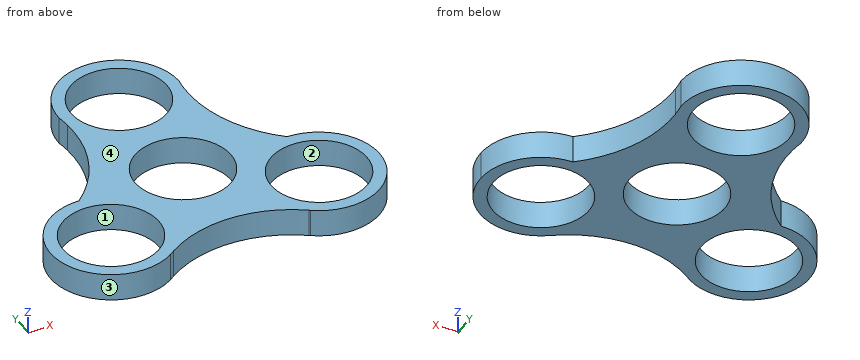
```python
from build123d import *

# Parameters (mm, degrees)
F0_R     = 11.049
F1_DEPTH = 6.35


with BuildPart() as f1:
    # F0 (on Top) → F1 (new body)
    with BuildSketch(Plane.XY):
        with BuildLine():
            ThreePointArc((24.1897099326, -0.0073616562), (15.9969747128, 11.215659094), (13.6372355628, 24.909042032))
            ThreePointArc((13.6372355628, 24.909042032), (-0.0068169573, 13.9700016632), (-13.6401871082, 24.9223526296))
            ThreePointArc((-13.6401871082, 24.9223526296), (-16.005456745, 11.2251220811), (-24.2066450876, 0.00241586))
            ThreePointArc((-24.2066450876, 0.00241586), (-14.3283633544, -4.0893024068), (-10.2366450876, -13.96758414))
            ThreePointArc((-10.2366450876, -13.96758414), (-11.6035855434, -19.9945062505), (-15.4369013691, -24.8419804502))
            ThreePointArc((-15.4369013691, -24.8419804502), (0.2894413219, -20.0870403352), (15.8966507841, -25.2195175864))
            ThreePointArc((15.8966507841, -25.2195175864), (10.9191820919, -9.6122739335), (24.1897099326, -0.0073616562))
        make_face()
        Circle(F0_R, mode=Mode.SUBTRACT)
        with BuildLine():
            ThreePointArc((-10.2366450876, -13.96758414), (-14.3283633544, -4.0893024068), (-24.2066450876, 0.00241586))
            ThreePointArc((-24.2066450876, 0.00241586), (-37.6059680769, -17.9196776899), (-16.6253454512, -25.7015006142))
            ThreePointArc((-16.6253454512, -25.7015006142), (-16.0368970517, -25.263757415), (-15.4369013691, -24.8419804502))
            ThreePointArc((-15.4369013691, -24.8419804502), (-11.6035855434, -19.9945062505), (-10.2366450876, -13.96758414))
        make_face()
        with Locations((-24.2066450876, -13.96758414)):
            Circle(F0_R, mode=Mode.SUBTRACT)
        with BuildLine():
            ThreePointArc((38.1597099326, -13.9773616562), (34.0679916658, -4.0990799231), (24.1897099326, -0.0073616562))
            ThreePointArc((24.1897099326, -0.0073616562), (10.9191820919, -9.6122739335), (15.8966507841, -25.2195175864))
            ThreePointArc((15.8966507841, -25.2195175864), (15.9879672376, -25.285462153), (16.0790108119, -25.3517829502))
            ThreePointArc((16.0790108119, -25.3517829502), (30.5871482201, -26.396447104), (38.1597099326, -13.9773616562))
        make_face()
        with Locations((24.1897099326, -13.9773616562)):
            Circle(F0_R, mode=Mode.SUBTRACT)
        with BuildLine():
            ThreePointArc((13.6372355628, 24.909042032), (13.7656925258, 26.4286847743), (13.97, 27.94))
            ThreePointArc((13.97, 27.94), (0, 41.91), (-13.97, 27.94))
            ThreePointArc((-13.97, 27.94), (-13.7675028866, 26.4352847759), (-13.6401871082, 24.9223526296))
            ThreePointArc((-13.6401871082, 24.9223526296), (-0.0068169573, 13.9700016632), (13.6372355628, 24.909042032))
        make_face()
        with Locations((0, 27.94)):
            Circle(F0_R, mode=Mode.SUBTRACT)
    extrude(amount=F1_DEPTH)


solid = f1.part
```
CAD build for the part. Positions are in the model's coordinates, mm. Face numbers are marked on the shaded views. Give positions to 0.01 mm unless a question says otherwise; leave off trailing zeros. Order: outer loops, then holes, each group sorted by start corner. A loop starts at its lowest first (then second) coordinate and runs counter-clockwise, first axis right, second up. Notation, with made-up numbers: M -32,-36 L 12,-36 A21 cw 12,-6 Z; hole C 37,-31 d2. An arc over 180 degrees is marked long. Put each result on its own line as item: value. Start each with the question number.
(1) Drill centre lines: line 1 along Y through (x, z) = (0, 2.25); line 2 along X through (y, z) = (-5.5, 4.5); line 3 along X through (y, z) = (-5, 2.5). Where is each one in solid material? Low to high.
(2) Saw through at A-A, the plane x = 0. Write the cut outline in (y, z), then the cut area to 3 significant figures.
(3) Mould opens along Y. For the marked faces 1, 2, 3 and 4 say: +Y half, -Y half, draft (parallel to the pull), parting line (faces both ways), or undercut.
(4) Saw through at C-C, the plane z = 1. Write the cut outline in (x, y).
(5) Saw through at B-B, the plane y = -23. Write the cut outline in (x, z), then the cut area to 3 significant figures.
(6) Flat gauge pins, fed straight in: pin 1 Ø13.5 at (x, y) = (0, 27.94) entering from -Z; pin 2 Ø2 at (x, z) = (4, 4) entering from +Y; pin 3 Ø1 at (y, z) = (7, 1.5) entering from -X. Where does each tip first touch, or does it go through?
(7) Saw through at D-D, the plane y = 24. Write the cut outline in (x, z), then the cut area to 3 significant figures.
Check result:
1. line 1: y = -20.09 to -11.05, 11.05 to 16.89, 38.99 to 41.91
1. line 2: x = -35.32 to -31.3, -17.11 to -9.58, 9.58 to 17.1, 31.28 to 35.29
1. line 3: x = -34.92 to -30.66, -17.75 to -9.85, 9.85 to 17.75, 30.63 to 34.89
2. outline: M -20.09,0 L -11.05,0 L -11.05,6.35 L -20.09,6.35 Z; M 11.05,0 L 16.89,0 L 16.89,6.35 L 11.05,6.35 Z; M 38.99,0 L 41.91,0 L 41.91,6.35 L 38.99,6.35 Z
2. area: 113 mm2
3. face 1: undercut
3. face 2: undercut
3. face 3: parting line
3. face 4: draft
4. outline: M -24.21,0 A13.97 ccw long -16.63,-25.7 A27.3 cw 15.9,-25.22 A27.3 cw 16.08,-25.35 A13.97 ccw long 24.19,-0.01 A30.48 cw 13.97,27.94 A13.97 ccw -13.97,27.94 A30.48 cw Z; hole C -24.21,-13.97 d22.1; hole C 0,0 d22.1; hole C 0,27.94 d22.1; hole C 24.19,-13.98 d22.1
5. outline: M -34.86,0 L -30.57,0 L -30.57,6.35 L -34.86,6.35 Z; M -17.84,0 L -12.31,0 L -12.31,6.35 L -17.84,6.35 Z; M 12.23,0 L 17.81,0 L 17.81,6.35 L 12.23,6.35 Z; M 30.57,0 L 34.86,0 L 34.86,6.35 L 30.57,6.35 Z
5. area: 125 mm2
6. pin 1: passes through
6. pin 2: stops at y = 41.58
6. pin 3: stops at x = -18.52
7. outline: M -13.6,0 L -10.32,0 L -10.32,6.35 L -13.6,6.35 Z; M 10.32,0 L 13.6,0 L 13.6,6.35 L 10.32,6.35 Z
7. area: 41.6 mm2
